Check sheet for the modelled part. Datum: model origin and axes. Units: mm. A direction names the side the tool comes from. Round coordinates to 2 decimals unless told otherwise and drop trailing zeros. Order: outer loops, then holes, each group sorted by start corner. A loop starts at its lowest first (then second) coordinate and runs counter-clockwise, first axis right, second up. Notation, with made-up numbers: M -30.75,10.25 L 14.25,10.25 A35 ccw 14.25,43.25 Z; hole C 57,-21 d9. An arc over 180 degrees is marked long. One line per item, written item: value. Start each with the question number.
(1) Cross-section at D-D, the plane x = 42. Enter the section's corners in (y, z).
(2) Access from +Z, -Z, +X, -X, +Y, -Y to the whole of each face (thin tool, end or side, straight path). Record for faces 1 (the face through (27.181, -12.005, 15.933)), 2 (the face through (10, 0, 13)), 3 (the face through (31.506, -2, 13)), 4 (the face through (0.437, -30, 14)), 5 (the face through (8.029, -30.941, 15.933)).
(3) Cross-section at C-C, the plane y = 5. Enter the section's corners in (x, z), and give its area (3 significant figures).
(4) Release check for a two-part mould opening along Y. For faces 6 (the face through (25, 46, 13)), 7 (the face through (25, 50, 13)), 8 (the face through (25, 17, 0)) record: released by +Y, released by -Y, zero draft, split by the parting line, or undercut.
(5) Depth check by flat-ended pin: pin 1 Ø8 at (x, z) = (26.5, 9) entering from -Y; pin 2 Ø15 at (x, z) = (44.5, 13) entering from -Y; pin 3 Ø1.2 at (x, y) = (25, 45) entering from +Z; pin 4 Ø1.5 at (y, z) = (-30.5, 14) entering from -X. Enter the tip coordinate at first touch or a pass-through.
(6) Cross-section at B-B, the plane z = 3. Enter the section's corners in (x, y).
(7) Thickness scan on L1, parallel to Y at x = 25, z = 17.5; L2, parallel to Y at x = 25, z = 12.25; L3, parallel to Y at x = 47, z = 8.25. Record the ranges inside material, lowest first.
(8) Cross-section at A-A, the plane y = 25. Enter the section's corners in (x, z), and give its area (3 significant figures).
from build123d import *

# Parameters (mm, degrees)
SKETCH1_W           = 50
SKETCH1_H           = 50
BOSS_EXTRUDE1_DEPTH = 25.4
SKETCH2_R           = 7.5
SKETCH2_R_2         = 1
CUT_EXTRUDE1_DEPTH  = 26.4
SKETCH3_W           = 11.506935687
SKETCH3_H           = 4.197505038
BOSS_EXTRUDE2_DEPTH = 25.4
SKETCH4_R           = 2.5


with BuildPart() as part:
    # Sketch1 → Boss-Extrude1 (new body)
    with BuildSketch(Plane.XY):
        with Locations((25, 25)):
            Rectangle(SKETCH1_W, SKETCH1_H)
    extrude(amount=BOSS_EXTRUDE1_DEPTH)

    # Sketch2 → Cut-Extrude1 (cut, through all)
    with BuildSketch(Plane.XY.offset(25.4)):
        with Locations((25, 25)):
            Circle(SKETCH2_R)
        with Locations((25, 45)):
            Circle(SKETCH2_R_2)
        with Locations((25, 5)):
            Circle(SKETCH2_R_2)
    extrude(amount=-CUT_EXTRUDE1_DEPTH, mode=Mode.SUBTRACT)

    # Sketch3 → Boss-Extrude2 (add)
    with BuildSketch(Plane.XY.offset(25.4)):
        with Locations((25.752790186, -2.098752519)):
            Rectangle(SKETCH3_W, SKETCH3_H)
    extrude(amount=-BOSS_EXTRUDE2_DEPTH)

    # Sweep1: sweep along a path in Sketch5
    with BuildLine(Plane(origin=(0, 0, 13.825315415), x_dir=(-1, 0, 0), z_dir=(0, 0, -1))) as sweep1_path:
        Line((-25.836773001, -4.197505038), (-25.836773001, -19.597505038))
        ThreePointArc((-25.836773001, -19.597505038), (-22.907840813, -26.66857285), (-15.836773001, -29.597505038))
        Line((-15.836773001, -29.597505038), (-0.436773001, -29.597505038))
    # Sketch4 → Sweep1 (sweep)
    with BuildSketch(Plane.XZ.offset(4.197505038)):
        with Locations((25.836773001, 13.825315415)):
            Circle(SKETCH4_R)
    sweep(path=sweep1_path.line)


solid = part.part
Values found:
1. outline: M 0,0 L 50,0 L 50,25.4 L 0,25.4 Z
2. face 1: none
2. face 2: +Z, -Z, -X
2. face 3: +Z, -Z, +X, -Y
2. face 4: +Z, -Z, -X, -Y
2. face 5: -X
3. outline: M 0,0 L 24,0 L 24,25.4 L 0,25.4 Z; M 26,0 L 50,0 L 50,25.4 L 26,25.4 Z
3. area: 1,220 mm^2
4. face 6: undercut
4. face 7: released by +Y
4. face 8: zero draft
5. pin 1: y = -28.16
5. pin 2: y = 0
5. pin 3: through
5. pin 4: x = 0.44
6. outline: M 0,0 L 20,0 L 20,-4.2 L 31.51,-4.2 L 31.51,0 L 50,0 L 50,50 L 0,50 Z; hole C 25,25 d15; hole C 25,5 d2; hole C 25,45 d2
7. L1: -4.2 to 4, 6 to 17.5, 32.5 to 44, 46 to 50
7. L2: -27.25 to 4, 6 to 17.5, 32.5 to 44, 46 to 50
7. L3: 0 to 50
8. outline: M 0,0 L 17.5,0 L 17.5,25.4 L 0,25.4 Z; M 32.5,0 L 50,0 L 50,25.4 L 32.5,25.4 Z
8. area: 889 mm^2
